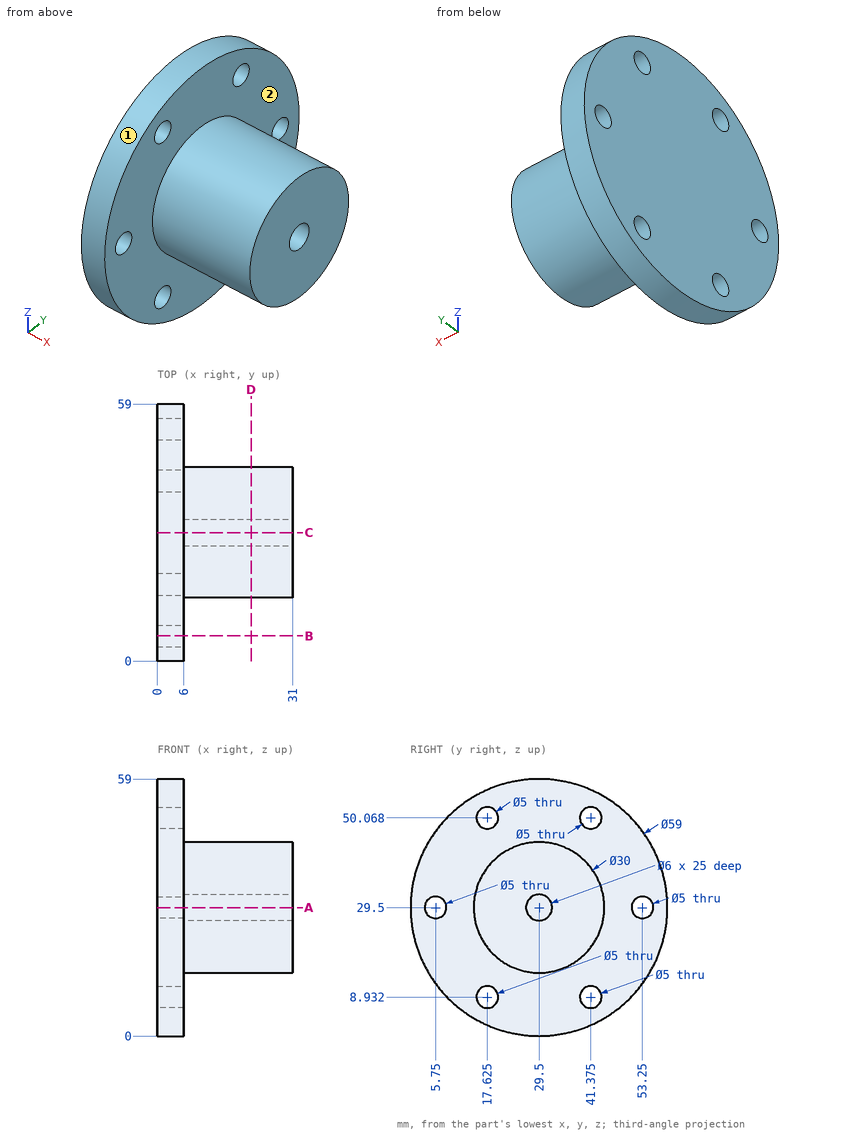
Here's the drawing with two shaded views (mm, measured from the low corner). I have some questions. A direction names the side the tool comes from. Coordinates: 2 decimals unless noted, no trailing zeros. Loops run counter-clockwise (first coordinate to the right, second up) from the corner with the lowest first, then second, coordinate; pieces in that order, holes last. Notation, with made-up numbers: (-34.75, 52.25) - (12.25, 52.25) arc R24 cw to (12.25, 66.25) - close; hole circle Ø4 at (24.5, -23.75). An arc over 180 degrees is marked (long way). Answer as CSV lines item,"result". Start each with the question number.
1) Suppose I cut it at B-B (y = 5.75). Please give me the cut outline in (x, z).
2) I need wall thicknesses on line 1 (Y direction, x = 18.75, z = 29.5); line 2 (Y direction, x = 3, z = 30); line 3 (X direction, y = 31.5, z = 31). Which ranges of each line are inside material? Lowest first, please. Write a range as from..to.
3) Suppose I cut it at D-D (x = 21.5). Please give me the cut outline in (y, z), plus the area to 3 significant figures.
4) For pin 1 (4 mm diameter, centred on x = 13.5, z = 32.5, fed in from +Y); pin 2 (8 mm diameter, centred on y = 41.38, z = 50.07, fed in from -X); pin 3 (5 mm diameter, centred on x = 4, y = 20, fed in from +Z); pin 4 (3 mm diameter, centred on y = 29, z = 29, fed in from +X), each with a flat end and sliding along its axis, tell me the tip position at first contact or that it passes through.
5) Suppose I cut it at C-C (y = 29.5). Please give me the cut outline in (x, z), plus the area to 3 significant figures.
6) Suppose I cut it at A-A (z = 29.5). Please give me the cut outline in (x, y).
7) Which directions (+Z, -Z, +X, -X, +Y, -Y) give clear straight access to the entire face, cutting with the end or side of a thin tool? Please do the marked faces 1 and 2.
Check result:
1,outline,"(0, 12) - (6, 12) - (6, 27) - (0, 27) - close; (0, 32) - (6, 32) - (6, 47) - (0, 47) - close"
2,line 1,"y = 14.5..26.5, 32.5..44.5"
2,line 2,"y = 0..3.3, 8.2..50.8, 55.7..59"
2,line 3,"x = 0..6"
3,outline,"circle Ø30 at (29.5, 29.5); hole circle Ø6 at (29.5, 29.5)"
3,area,"679 mm²"
4,pin 1,"stops at y = 44.47"
4,pin 2,"stops at x = 0"
4,pin 3,"stops at z = 58.16"
4,pin 4,"stops at x = 6"
5,outline,"(0, 0) - (6, 0) - (6, 14.5) - (31, 14.5) - (31, 26.5) - (6, 26.5) - (6, 32.5) - (31, 32.5) - (31, 44.5) - (6, 44.5) - (6, 59) - (0, 59) - close"
5,area,"954 mm²"
6,outline,"(0, 0) - (6, 0) - (6, 3.25) - (0, 3.25) - close; (0, 8.25) - (6, 8.25) - (6, 14.5) - (31, 14.5) - (31, 26.5) - (6, 26.5) - (6, 32.5) - (31, 32.5) - (31, 44.5) - (6, 44.5) - (6, 50.75) - (0, 50.75) - close; (0, 55.75) - (6, 55.75) - (6, 59) - (0, 59) - close"
7,face 1,"+X, -X"
7,face 2,"+X"
